Read the model definition and answer for the solid it produces. Units are mm, in the model's axes. Face numbers are marked on the shaded views. A direction names the side the tool comes from. Coordinates: 2 decimals unless noted, no trailing zeros. Loops run counter-clockwise (first coordinate to the right, second up) from the corner with the lowest first, then second, coordinate; pieces in that order, holes last. Notation, with made-up numbers: (58, 62) -> (76, 62) arc R18 ccw to (76, 95) -> close; hole circle Ø9 at (57.5, 77). An arc over 180 degrees is marked (long way). Answer in a Markdown table with one row per item.
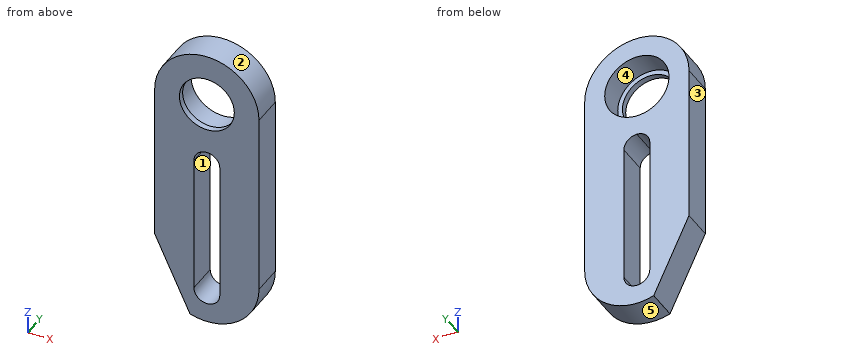
```python
from build123d import *

# Parameters (mm, degrees)
SKETCH1_R           = 6.65
SKETCH1_R_2         = 4.1
BOSS_EXTRUDE1_DEPTH = 4
SKETCH2_R           = 4.1
BOSS_EXTRUDE2_DEPTH = 0.8
SKETCH3_R           = 3.5
CUT_EXTRUDE1_DEPTH  = 1.8
CUT_EXTRUDE2_DEPTH  = 5


with BuildPart() as part:
    # Sketch1 → Boss-Extrude1 (new body)
    with BuildSketch(Plane(origin=(0, 0, 0), x_dir=(1, 0, 0), z_dir=(0, 1, 0))):
        with BuildLine():
            Line((-6.65, 23.5), (-6.65, 0))
            ThreePointArc((-6.65, 0), (-4.702260096, 4.702260094), (-2e-09, 6.65))
            ThreePointArc((-2e-09, 6.65), (4.702260094, 4.702260096), (6.65, 0))
            Line((6.65, 0), (6.65, 23.5))
            ThreePointArc((6.65, 23.5), (0, 30.15), (-6.65, 23.5))
        make_face()
        with BuildLine():
            ThreePointArc((1.65, 8.3), (1.166726188, 7.13327381), (-2e-09, 6.65))
            ThreePointArc((-2e-09, 6.65), (-1.16672619, 7.133273812), (-1.65, 8.3))
            Line((-1.65, 8.3), (-1.65, 26))
            ThreePointArc((-1.65, 26), (0, 27.65), (1.65, 26))
            Line((1.65, 26), (1.65, 8.3))
        make_face(mode=Mode.SUBTRACT)
        Circle(SKETCH1_R)
        Circle(SKETCH1_R_2, mode=Mode.SUBTRACT)
    extrude(amount=BOSS_EXTRUDE1_DEPTH)

    # Sketch2 → Boss-Extrude2 (add)
    with BuildSketch(Plane(origin=(0, 0, 0), x_dir=(1, 0, 0), z_dir=(0, 1, 0))):
        Circle(SKETCH2_R)
    extrude(amount=BOSS_EXTRUDE2_DEPTH)

    # Sketch3 → Cut-Extrude1 (cut, through all)
    with BuildSketch(Plane(origin=(0, 0.8, 0), x_dir=(1, 0, 0), z_dir=(0, 1, 0))):
        Circle(SKETCH3_R)
    extrude(amount=-CUT_EXTRUDE1_DEPTH, mode=Mode.SUBTRACT)

    # Sketch4 → Cut-Extrude2 (cut, through all)
    with BuildSketch(Plane.XZ):
        with BuildLine():
            Line((-6.65, -20.142571947), (-2.15, -29.792853089))
            ThreePointArc((-2.15, -29.792853089), (-5.409251335, -27.368139087), (-6.65, -23.5))
            Line((-6.65, -23.5), (-6.65, -20.142571947))
        make_face()
    extrude(amount=-CUT_EXTRUDE2_DEPTH, mode=Mode.SUBTRACT)


solid = part.part
```
1. The mould has two halves that part along Z. Classify the marked faces 3, 4 and 5: pulls with the +Z half, pulls with the -Z half, needs draft (parallel to the pull), parting line crosses it, or undercut.
A:
| item | result |
|---|---|
| face 3 | needs draft |
| face 4 | undercut |
| face 5 | pulls with the -Z half |
2. A cutting plane is placed at C-C on z = -7. Give the vertices of the cut face in (x, y).
A:
| item | result |
|---|---|
| outline | (-6.65, 0) -> (-1.02, 0) -> (-1.02, 4) -> (-6.65, 4) -> close; (1.02, 0) -> (6.65, 0) -> (6.65, 4) -> (1.02, 4) -> close |
3. A tool of negligible diameter and unlimited length cuts with its end or side. For the marked faces 1 and 2, from which of +Z, -Z, +X, -X, +Y, -Y can it reach the whole face along a straight path? Write none if from no direction.
A:
| item | result |
|---|---|
| face 1 | +Y, -Y |
| face 2 | +Z, +Y, -Y |
4. Given pin 1 Ø6.5 at (x, z) = (0, 0) entering from +Y; pin 2 Ø4 at (x, z) = (1, -1.5) entering from +Y, each flat-ended and moving along its own axis, determine where each tip first touches the part or whether it passes through.
A:
| item | result |
|---|---|
| pin 1 | passes through |
| pin 2 | stops at y = 0.8 |
5. A cutting plane is placed at A-A on y = 0.45. Give the vertices of the cut face in (x, z), and give its area (3 significant figures).
A:
| item | result |
|---|---|
| outline | (-6.65, -20.14) -> (-2.15, -29.79) arc R6.65 ccw to (6.65, -23.5) -> (6.65, 0) arc R6.65 ccw to (-6.65, 0) -> close; hole circle Ø7 at (0, 0); hole (-1.65, -26) arc R1.65 ccw to (1.65, -26) -> (1.65, -8.3) arc R1.65 ccw to (-1.65, -8.3) -> close |
| area | 332 mm2 |
6. A cutting plane is placed at B-B on z = 1.5. Give the vertices of the cut face in (x, y).
A:
| item | result |
|---|---|
| outline | (-6.48, 0) -> (-3.16, 0) -> (-3.16, 0.8) -> (-3.82, 0.8) -> (-3.82, 4) -> (-6.48, 4) -> close; (3.16, 0) -> (6.48, 0) -> (6.48, 4) -> (3.82, 4) -> (3.82, 0.8) -> (3.16, 0.8) -> close |
7. Find the intervals of material crossed by probe 1 along Z at (x, y) = (0, 1.7); probe 2 along Z at (x, y) = (0, 0.5); probe 3 along X at (y, z) = (0.5, 0), in increasing order.
A:
| item | result |
|---|---|
| probe 1 | z = -30.15 to -27.65, -6.65 to -4.1, 4.1 to 6.65 |
| probe 2 | z = -30.15 to -27.65, -6.65 to -3.5, 3.5 to 6.65 |
| probe 3 | x = -6.65 to -3.5, 3.5 to 6.65 |
